Geometry check sheet. Reference: the model listing, model coordinates, mm. A direction names the side the tool comes from. Round coordinates to 2 decimals unless told otherwise and drop trailing zeros. Loops run counter-clockwise (first coordinate to the right, second up) from the corner with the lowest first, then second, coordinate; pieces in that order, holes last.
```python
from build123d import *

# Parameters (mm, degrees)
F1_DEPTH = 6
F2_W     = 9
F2_H     = 6
F3_DEPTH = 13.0652172513


with BuildPart() as f1:
    # F0 (on Right) → F1 (new body, symmetric)
    with BuildSketch(Plane.YZ):
        Polygon((-29.184781258, 0), (8.7065214151, 0), (8.7065214151, 9), (5.8369566332, 9), (-3.3586958362, 1.5), (-29.184781258, 1.5), align=None)
    extrude(amount=F1_DEPTH, both=True)

    # F2 (on face) → F3 (cut, up to face)
    with BuildSketch(Plane(origin=(0, 8.7065214151, 0), x_dir=(-1, 0, 0), z_dir=(0, 1, 0))):
        with Locations((0, 4.5)):
            Rectangle(F2_W, F2_H)
    extrude(amount=-F3_DEPTH, mode=Mode.SUBTRACT)


solid = f1.part
```
1) Mould release check, pull along Z, two halves, no side actions. Record for faces 1 (the face through (0, -11, 0)), 2 (the face through (6, -2, 2)), 3 (the face through (-4.5, 4, 4)), 4 (the face through (0.084, 4.369, 7.802)): +Z half, -Z half, draft (parallel to the pull), parting line (faces both ways), or undercut.
Report:
face 1: -Z half
face 2: draft
face 3: undercut
face 4: +Z half
2) Access from +Z, -Z, +X, -X, +Y, -Y to the whole of each face (thin tool, end or side, straight path). Record for faces 5 (the face through (-6, -2, 2)), 6 (the face through (4.5, 4, 4)).
Report:
face 5: +Z, -Z, -X, +Y, -Y
face 6: +Y, -Y
3) Sectioned sample at D-D, the plane x = 5.25. Record the cut outline in (y, z).
Report:
outline: (-29.18, 0) - (8.71, 0) - (8.71, 9) - (5.84, 9) - (-3.36, 1.5) - (-29.18, 1.5) - close
4) Scan lines: line 1 along X through (y, z) = (7.5, 2.25); line 2 along Z through (x, y) = (4, 5); line 3 along Z through (x, y) = (-1, -9.5). Record each from-to range of solid material in increasing order.
Report:
line 1: x = -6 to -4.5, 4.5 to 6
line 2: z = 0 to 1.5, 7.5 to 8.32
line 3: z = 0 to 1.5
5) Gauge pin test, flat end, axial feed: pin 1 (6 mm diameter, centred on x = -1, y = -6.5, fed in from +Z). Record the tip position at first contact, or that the pin passes through.
Report:
pin 1: stops at z = 1.5
6) Sectioned sample at A-A, the plane z = 6.75. Record the cut outline in (x, y), then the cut area to 3 significant figures.
Report:
outline: (-6, 3.08) - (-4.5, 3.08) - (-4.5, 8.71) - (-6, 8.71) - close; (4.5, 3.08) - (6, 3.08) - (6, 8.71) - (4.5, 8.71) - close
area: 16.9 mm2
7) Sectioned sample at B-B, the plane x = -1.5. Record the cut outline in (y, z).
Report:
outline: (-29.18, 0) - (8.71, 0) - (8.71, 1.5) - (-29.18, 1.5) - close; (4, 7.5) - (8.71, 7.5) - (8.71, 9) - (5.84, 9) - close
8) Sectioned sample at C-C, the plane y = -18.5. Record the cut outline in (x, z).
Report:
outline: (-6, 0) - (6, 0) - (6, 1.5) - (-6, 1.5) - close
